Geometry: final body of the model. Coordinates: model frame, mm. Give positions to 0.01 mm unless a question says otherwise; leave off trailing zeros. Write each loop counter-clockwise with the first axis right and the second up, starting at its lowest first coordinate (ties: lowest second). Pieces come first, ordered by that corner, then holes.
```python
from build123d import *

# Parameters (mm, degrees)
SKETCH1_W           = 260
SKETCH1_H           = 600
SKETCH1_R           = 1.6
SKETCH1_W_2         = 100
SKETCH1_H_2         = 320
BOSS_EXTRUDE1_DEPTH = 3.175
FILLET1_R           = 3


with BuildPart() as part:
    # Sketch1 → Boss-Extrude1 (new body)
    with BuildSketch(Plane(origin=(0, 0, 0), x_dir=(1, 0, 0), z_dir=(0, 1, 0))):
        Rectangle(SKETCH1_W, SKETCH1_H)
        with Locations(Location((120, 290, 0), (0, 0, 270))):
            Circle(SKETCH1_R, mode=Mode.SUBTRACT)
        with Locations(Location((120, 232, 0), (0, 0, 270))):
            Circle(SKETCH1_R, mode=Mode.SUBTRACT)
        with Locations(Location((120, 174, 0), (0, 0, 270))):
            Circle(SKETCH1_R, mode=Mode.SUBTRACT)
        with Locations(Location((120, 116, 0), (0, 0, 270))):
            Circle(SKETCH1_R, mode=Mode.SUBTRACT)
        with Locations(Location((120, 58, 0), (0, 0, 270))):
            Circle(SKETCH1_R, mode=Mode.SUBTRACT)
        with Locations(Location((120, 0, 0), (0, 0, 270))):
            Circle(SKETCH1_R, mode=Mode.SUBTRACT)
        with Locations(Location((120, -58, 0), (0, 0, 270))):
            Circle(SKETCH1_R, mode=Mode.SUBTRACT)
        with Locations(Location((120, -116, 0), (0, 0, 270))):
            Circle(SKETCH1_R, mode=Mode.SUBTRACT)
        with Locations(Location((120, -174, 0), (0, 0, 270))):
            Circle(SKETCH1_R, mode=Mode.SUBTRACT)
        with Locations(Location((120, -232, 0), (0, 0, 270))):
            Circle(SKETCH1_R, mode=Mode.SUBTRACT)
        with Locations(Location((120, -290, 0), (0, 0, 270))):
            Circle(SKETCH1_R, mode=Mode.SUBTRACT)
        with Locations(Location((-120, 232, 0), (0, 0, 90))):
            Circle(SKETCH1_R, mode=Mode.SUBTRACT)
        with Locations(Location((-120, -290, 0), (0, 0, 90))):
            Circle(SKETCH1_R, mode=Mode.SUBTRACT)
        with Locations(Location((-120, -232, 0), (0, 0, 90))):
            Circle(SKETCH1_R, mode=Mode.SUBTRACT)
        with Locations(Location((-120, -174, 0), (0, 0, 90))):
            Circle(SKETCH1_R, mode=Mode.SUBTRACT)
        with Locations(Location((-120, -116, 0), (0, 0, 90))):
            Circle(SKETCH1_R, mode=Mode.SUBTRACT)
        with Locations(Location((-120, -58, 0), (0, 0, 90))):
            Circle(SKETCH1_R, mode=Mode.SUBTRACT)
        with Locations(Location((-120, 0, 0), (0, 0, 90))):
            Circle(SKETCH1_R, mode=Mode.SUBTRACT)
        with Locations(Location((-120, 58, 0), (0, 0, 90))):
            Circle(SKETCH1_R, mode=Mode.SUBTRACT)
        with Locations(Location((-120, 116, 0), (0, 0, 90))):
            Circle(SKETCH1_R, mode=Mode.SUBTRACT)
        with Locations(Location((-120, 174, 0), (0, 0, 90))):
            Circle(SKETCH1_R, mode=Mode.SUBTRACT)
        with Locations(Location((-120, 290, 0), (0, 0, 90))):
            Circle(SKETCH1_R, mode=Mode.SUBTRACT)
        with Locations(Location((112, 235, 0), (0, 0, 270))):
            Circle(SKETCH1_R, mode=Mode.SUBTRACT)
        with Locations(Location((-112, 235, 0), (0, 0, 90))):
            Circle(SKETCH1_R, mode=Mode.SUBTRACT)
        with Locations(Location((112, -235, 0), (0, 0, 90))):
            Circle(SKETCH1_R, mode=Mode.SUBTRACT)
        with Locations(Location((-112, -235, 0), (0, 0, 270))):
            Circle(SKETCH1_R, mode=Mode.SUBTRACT)
        with Locations(Location((104, 290, 0), (0, 0, 270))):
            Circle(SKETCH1_R, mode=Mode.SUBTRACT)
        with Locations(Location((104, 232, 0), (0, 0, 270))):
            Circle(SKETCH1_R, mode=Mode.SUBTRACT)
        with Locations(Location((104, 174, 0), (0, 0, 270))):
            Circle(SKETCH1_R, mode=Mode.SUBTRACT)
        with Locations(Location((104, 116, 0), (0, 0, 270))):
            Circle(SKETCH1_R, mode=Mode.SUBTRACT)
        with Locations(Location((104, 58, 0), (0, 0, 270))):
            Circle(SKETCH1_R, mode=Mode.SUBTRACT)
        with Locations(Location((104, 0, 0), (0, 0, 270))):
            Circle(SKETCH1_R, mode=Mode.SUBTRACT)
        with Locations(Location((104, -58, 0), (0, 0, 270))):
            Circle(SKETCH1_R, mode=Mode.SUBTRACT)
        with Locations(Location((104, -116, 0), (0, 0, 270))):
            Circle(SKETCH1_R, mode=Mode.SUBTRACT)
        with Locations(Location((104, -174, 0), (0, 0, 270))):
            Circle(SKETCH1_R, mode=Mode.SUBTRACT)
        with Locations(Location((104, -232, 0), (0, 0, 270))):
            Circle(SKETCH1_R, mode=Mode.SUBTRACT)
        with Locations(Location((104, -290, 0), (0, 0, 270))):
            Circle(SKETCH1_R, mode=Mode.SUBTRACT)
        with Locations(Location((-104, -290, 0), (0, 0, 90))):
            Circle(SKETCH1_R, mode=Mode.SUBTRACT)
        with Locations(Location((-104, -174, 0), (0, 0, 90))):
            Circle(SKETCH1_R, mode=Mode.SUBTRACT)
        with Locations(Location((-104, -116, 0), (0, 0, 90))):
            Circle(SKETCH1_R, mode=Mode.SUBTRACT)
        with Locations(Location((-104, -58, 0), (0, 0, 90))):
            Circle(SKETCH1_R, mode=Mode.SUBTRACT)
        with Locations(Location((-104, 0, 0), (0, 0, 90))):
            Circle(SKETCH1_R, mode=Mode.SUBTRACT)
        with Locations(Location((-104, 58, 0), (0, 0, 90))):
            Circle(SKETCH1_R, mode=Mode.SUBTRACT)
        with Locations(Location((-104, 116, 0), (0, 0, 90))):
            Circle(SKETCH1_R, mode=Mode.SUBTRACT)
        with Locations(Location((-104, 174, 0), (0, 0, 90))):
            Circle(SKETCH1_R, mode=Mode.SUBTRACT)
        with Locations(Location((-104, 232, 0), (0, 0, 90))):
            Circle(SKETCH1_R, mode=Mode.SUBTRACT)
        with Locations(Location((-104, 290, 0), (0, 0, 90))):
            Circle(SKETCH1_R, mode=Mode.SUBTRACT)
        with Locations(Location((-104, -232, 0), (0, 0, 90))):
            Circle(SKETCH1_R, mode=Mode.SUBTRACT)
        with Locations(Location((112, 0, 0), (0, 0, 270))):
            Circle(SKETCH1_R, mode=Mode.SUBTRACT)
        with Locations(Location((-112, 0, 0), (0, 0, 90))):
            Circle(SKETCH1_R, mode=Mode.SUBTRACT)
        with Locations(Location((-50, -290, 0), (0, 0, 270))):
            Circle(SKETCH1_R, mode=Mode.SUBTRACT)
        with Locations(Location((-50, -266, 0), (0, 0, 270))):
            Circle(SKETCH1_R, mode=Mode.SUBTRACT)
        with Locations(Location((50, -266, 0), (0, 0, 90))):
            Circle(SKETCH1_R, mode=Mode.SUBTRACT)
        with Locations(Location((50, -290, 0), (0, 0, 90))):
            Circle(SKETCH1_R, mode=Mode.SUBTRACT)
        with Locations(Location((-26, -290, 0), (0, 0, 90))):
            Circle(SKETCH1_R, mode=Mode.SUBTRACT)
        with Locations(Location((-26, -266, 0), (0, 0, 90))):
            Circle(SKETCH1_R, mode=Mode.SUBTRACT)
        with Locations(Location((26, -290, 0), (0, 0, 270))):
            Circle(SKETCH1_R, mode=Mode.SUBTRACT)
        with Locations(Location((26, -266, 0), (0, 0, 270))):
            Circle(SKETCH1_R, mode=Mode.SUBTRACT)
        with Locations(Location((-72, 290, 0), (0, 0, 90))):
            Circle(SKETCH1_R, mode=Mode.SUBTRACT)
        with Locations(Location((-72, 232, 0), (0, 0, 90))):
            Circle(SKETCH1_R, mode=Mode.SUBTRACT)
        with Locations(Location((-40, 290, 0), (0, 0, 90))):
            Circle(SKETCH1_R, mode=Mode.SUBTRACT)
        with Locations(Location((-40, 232, 0), (0, 0, 90))):
            Circle(SKETCH1_R, mode=Mode.SUBTRACT)
        with Locations(Location((-8, 290, 0), (0, 0, 90))):
            Circle(SKETCH1_R, mode=Mode.SUBTRACT)
        with Locations(Location((-8, 232, 0), (0, 0, 90))):
            Circle(SKETCH1_R, mode=Mode.SUBTRACT)
        with Locations(Location((24, 290, 0), (0, 0, 90))):
            Circle(SKETCH1_R, mode=Mode.SUBTRACT)
        with Locations(Location((24, 232, 0), (0, 0, 90))):
            Circle(SKETCH1_R, mode=Mode.SUBTRACT)
        with Locations(Location((56, 290, 0), (0, 0, 90))):
            Circle(SKETCH1_R, mode=Mode.SUBTRACT)
        with Locations(Location((56, 232, 0), (0, 0, 90))):
            Circle(SKETCH1_R, mode=Mode.SUBTRACT)
        with Locations(Location((88, 290, 0), (0, 0, 90))):
            Circle(SKETCH1_R, mode=Mode.SUBTRACT)
        with Locations(Location((88, 232, 0), (0, 0, 90))):
            Circle(SKETCH1_R, mode=Mode.SUBTRACT)
        with Locations(Location((-12, -251, 0), (0, 0, 270))):
            Circle(SKETCH1_R, mode=Mode.SUBTRACT)
        with Locations(Location((-2, -251, 0), (0, 0, 270))):
            Circle(SKETCH1_R, mode=Mode.SUBTRACT)
        with Locations(Location((-12, -211, 0), (0, 0, 90))):
            Circle(SKETCH1_R, mode=Mode.SUBTRACT)
        with Locations(Location((-2, -211, 0), (0, 0, 90))):
            Circle(SKETCH1_R, mode=Mode.SUBTRACT)
        with Locations((0, 40)):
            Rectangle(SKETCH1_W_2, SKETCH1_H_2, mode=Mode.SUBTRACT)
    extrude(amount=BOSS_EXTRUDE1_DEPTH)

    # Fillet1
    fillet1_edges = [part.edges().sort_by_distance(p)[0] for p in [
        (50, 1.5875, 120),
        (50, 1.5875, -200),
        (-50, 1.5875, -200),
        (-50, 1.5875, 120),
        (130, 1.5875, 300),
        (-130, 1.5875, 300),
        (-130, 1.5875, -300),
        (130, 1.5875, -300),
    ]]
    fillet(fillet1_edges, radius=FILLET1_R)


solid = part.part
```
Item 1: Section B-B, the plane y = 1.85. State how many separate pieces and enclosed holes the cut face has, plus the area to 3 significant figures.
Found:
separate pieces: 1
enclosed holes: 75
area: 123,000 mm2
Item 2: Line query: L1, parallel to X at y = 1.1, z = 266; L2, parallel to X at y = 0.7, z = 58; L3, parallel to Z at x = 88, y = 1.15. Output: solid intervals per line, ascending.
Found:
L1: x = -130 to -51.6, -48.4 to -27.6, -24.4 to 24.4, 27.6 to 48.4, 51.6 to 130
L2: x = -130 to -121.6, -118.4 to -105.6, -102.4 to -50, 50 to 102.4, 105.6 to 118.4, 121.6 to 130
L3: z = -300 to -291.6, -288.4 to -233.6, -230.4 to 300
Item 3: Section A-A, the plane z = -94. Return the cut outline in (x, y) (3 decimals).
Found:
outline: (-130, 0) - (-50, 0) - (-50, 3.175) - (-130, 3.175) - close; (50, 0) - (130, 0) - (130, 3.175) - (50, 3.175) - close
Item 4: Pin query (flat end, axial travel): pin 1 Ø5 at (x, z) = (104, 232) entering from +Y (3 decimals). Return the tip coordinate at first contact, or that it passes through.
Found:
pin 1: stops at y = 3.175
